from build123d import *

# Parameters (mm, degrees)
SKETCH1_R           = 1.6
BOSS_EXTRUDE1_DEPTH = 4
FILLET1_R           = 10


with BuildPart() as part:
    # Sketch1 → Boss-Extrude1 (new body)
    with BuildSketch(Plane(origin=(0, 0, 0), x_dir=(0, 0, -1), z_dir=(1, 0, 0))):
        with BuildLine():
            Line((3.594627394, 0), (6.26129406, 0))
            ThreePointArc((6.26129406, 0), (7.688720424, 0.447573637), (8.60504406, 1.630036818))
            Line((8.60504406, 1.630036818), (16.138282763, 21.925181005))
            Line((16.138282763, 21.925181005), (20.42668985, 26.002896629))
            Line((20.42668985, 26.002896629), (50.91386883, 38.739566173))
            Line((50.91386883, 38.739566173), (68.844719883, 38.977888478))
            Line((68.844719883, 38.977888478), (68.844719883, 53.977888478))
            Line((68.844719883, 53.977888478), (55.845867993, 53.805118299))
            Line((55.845867993, 53.805118299), (18.937282625, 38.385769218))
            Line((18.937282625, 38.385769218), (11.690435574, 31.494963182))
            Line((11.690435574, 31.494963182), (1.250877394, 3.369963182))
            ThreePointArc((1.250877394, 3.369963182), (1.54220103, 1.072573637), (3.594627394, 0))
        make_face()
        with Locations((64.344719883, 50.977888478)):
            Circle(SKETCH1_R, mode=Mode.SUBTRACT)
        with Locations((4.927960727, 3)):
            Circle(SKETCH1_R, mode=Mode.SUBTRACT)
        with Locations((18.016916415, 30.611068767)):
            Circle(SKETCH1_R, mode=Mode.SUBTRACT)
        with Locations((37.879973994, 39.796930611)):
            Circle(SKETCH1_R, mode=Mode.SUBTRACT)
        with Locations((64.340323045, 41.977889552)):
            Circle(SKETCH1_R, mode=Mode.SUBTRACT)
    extrude(amount=BOSS_EXTRUDE1_DEPTH)

    # Fillet1
    fillet1_edges = [part.edges().sort_by_distance(p)[0] for p in [
        (2, 21.925181005, -16.138282763),
        (2, 26.002896629, -20.42668985),
        (2, 38.739566173, -50.91386883),
        (2, 53.805118299, -55.845867993),
        (2, 38.385769218, -18.937282625),
        (2, 31.494963182, -11.690435574),
    ]]
    fillet(fillet1_edges, radius=FILLET1_R)


solid = part.part
Here's how the part is built. I have some questions about the finished solid (model axes, mm). Give positions to 0.01 mm unless a question says otherwise; leave off trailing zeros. Order: outer loops, then holes, each group sorted by start corner. A loop starts at its lowest first (then second) coordinate and runs counter-clockwise, first axis right, second up. Notation, with made-up numbers: M -26,2.25 L -1,2.25 A12 ccw -1,10.25 Z; hole C -33.5,11.25 d5. An arc over 180 degrees is marked long. Answer as a JSON object with one key per item and string values. Group by question number.
1) We'd pull the mould along Z, two halves only. Please class faces 1 (the flat face through (0, 33, -35)), 2 (the cylindrical face through (1.972, 49.416, -63.998)), 3 (the flat face through (1.972, 35.132, -15.515)): pulls with the +Z half, pulls with the -Z half, needs draft (parallel to the pull), parting line crosses it, or undercut.
2) Suppose I cut it at B-B, the plane y = 28. Write out the boundary of the cut face in (x, z), plus the area to 3 significant figures.
3) Suppose I cut it at A-A, the plane x = 1.2. Write out the boundary of the cut face in (y, z), plus the area to 3 significant figures.
4) I'm going to push flat-ended pins straight in: pin 1 Ø12 at (y, z) = (34, -52) entering from -X; pin 2 Ø3 at (y, z) = (30.61, -18.02) entering from -X; pin 3 Ø1.5 at (x, z) = (2.5, -28) entering from -Y; pin 4 Ø1.5 at (x, z) = (1.5, -31) entering from +Y. Where does each tip first touch, or does it pass through?
5) Please list where these lines run through material, in increasing order: L1, parallel to Z at x = 3.25, y = 51.5; L2, parallel to Y at x = 0.25, z = -24; L3, parallel to Y at x = 0.7, z = -19. Write a range as [from, to].
6) Suppose I cut it at C-C, the plane z = -32. Write out the boundary of the cut face in (x, y).
Results found:
{
 "1": {"face 1": "needs draft", "face 2": "undercut", "face 3": "pulls with the +Z half"},
 "2": {"outline": "M 0,-25.21 L 4,-25.21 L 4,-10.39 L 0,-10.39 Z", "area": "59.3 mm²"},
 "3": {"outline": "M 0,-6.26 A2.5 ccw 1.63,-8.61 L 19.75,-15.33 A10 cw 23.52,-17.82 L 24.73,-19.09 A10 cw 26.71,-22.13 L 37.99,-49.13 A10 cw 38.77,-52.85 L 38.98,-68.84 L 53.98,-68.84 L 53.83,-57.78 A10 ccw 53.06,-54.06 L 39.1,-20.64 A10 ccw 37.12,-17.6 L 33.09,-13.37 A10 ccw 29.32,-10.88 L 3.37,-1.25 A2.5 ccw 0,-3.59 Z; hole C 3,-4.93 d3.2; hole C 30.61,-18.02 d3.2; hole C 39.8,-37.88 d3.2; hole C 41.98,-64.34 d3.2; hole C 50.98,-64.34 d3.2", "area": "920 mm²"},
 "4": {"pin 1": "x = 0", "pin 2": "through", "pin 3": "y = 28.85", "pin 4": "y = 43.74"},
 "5": {"L1": "[-68.84, -65.86], [-62.83, -50.33]", "L2": "[27.5, 40.5]", "L3": "[24.65, 29.35], [31.87, 38.23]"},
 "6": {"outline": "M 0,30.84 L 4,30.84 L 4,43.84 L 0,43.84 Z"}
}
